Source: CAD feature listing. Evaluate the final solid. Frame: model axes, mm. A direction names the side the tool comes from. Coordinates: 2 decimals unless noted, no trailing zeros. Order: outer loops, then holes, each group sorted by start corner. A loop starts at its lowest first (then second) coordinate and runs counter-clockwise, first axis right, second up. Notation, with made-up numbers: (36, -5) -> (54, -5) arc R22 ccw to (54, 24) -> close; hole circle Ø6 at (31.25, 70.25). An arc over 180 degrees is marked (long way). Write item = value, one per line. Start each with the question number.
Item 1: Set-up query: faces 1 (the flat face through (-62, 23, 2)), 2 (the flat face through (0, 9, 2)). Return all of +Z, -Z, +X, -X, +Y, -Y with unobstructed straight access to the full face (end or side cutting, diameter ignored); none if empty.
Item 2: Section query B-B (y = 26). Output: boundary loops of the cut face in (x, z), then the cut area to 3 significant figures.
Item 3: Section query C-C (x = -29). Output: boundary loops of the cut face in (y, z), then the cut area to 3 significant figures.
Item 4: Section query A-A (z = 2.25). Output: boundary loops of the cut face in (x, y).
Item 5: Ray query, line 1 along Y through (x, z) = (-30, 4.05); line 2 along X through (y, z) = (20.5, 3.3). Return the intervals inside material, ascending. Write a range as [from, to].
Item 6: Contact query for a flat-ended pin moving along its axis: pin 1 (3 mm diameter, centred on y = 13, z = 0.5, fed in from +X). Output: stop coordinate, or through.
```python
from build123d import *

# Parameters (mm, degrees)
BOSS_EXTRU_1_DEPTH = 5


with BuildPart() as part:
    # Esquisse1 → Boss.-Extru.1 (new body)
    with BuildSketch(Plane.XY):
        with BuildLine():
            Line((-2, 0), (-67, 0))
            ThreePointArc((-67, 0), (-68.414213562, 0.585786438), (-69, 2))
            Line((-69, 2), (-69, 27.5))
            ThreePointArc((-69, 27.5), (-67.974873734, 29.974873734), (-65.5, 31))
            Line((-65.5, 31), (-64, 31))
            ThreePointArc((-64, 31), (-62.585786438, 30.414213562), (-62, 29))
            Line((-62, 29), (-62, 17))
            ThreePointArc((-62, 17), (-61.414213562, 15.585786438), (-60, 15))
            Line((-60, 15), (0, 15))
            Line((0, 15), (0, 2))
            ThreePointArc((0, 2), (-0.585786438, 0.585786438), (-2, 0))
        make_face()
    extrude(amount=BOSS_EXTRU_1_DEPTH)


solid = part.part
```
Computed:
q1.face_1 = +Z, -Z, +X, +Y
q1.face_2 = +Z, -Z, +X, +Y, -Y
q2.outline = (-69, 0) -> (-62, 0) -> (-62, 5) -> (-69, 5) -> close
q2.area = 35.0 mm^2
q3.outline = (0, 0) -> (15, 0) -> (15, 5) -> (0, 5) -> close
q3.area = 75.0 mm^2
q4.outline = (-69, 2) arc R2 ccw to (-67, 0) -> (-2, 0) arc R2 ccw to (0, 2) -> (0, 15) -> (-60, 15) arc R2 cw to (-62, 17) -> (-62, 29) arc R2 ccw to (-64, 31) -> (-65.5, 31) arc R3.5 ccw to (-69, 27.5) -> close
q5.line_1 = [0, 15]
q5.line_2 = [-69, -62]
q6.pin_1 = 0
